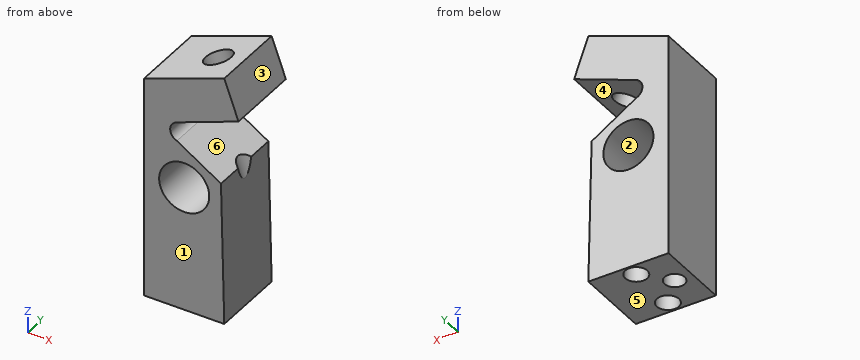
from build123d import *

# Parameters (mm, degrees)
F0_R     = 5
F1_DEPTH = 15
F3_D     = 5.5
F3_DEPTH = 50
F3_TIP   = 1.6523667023
F5_D     = 4.4
F5_DEPTH = 8
F5_TIP   = 1.3218933619
F6_R     = 2
F7_DEPTH = 5


with BuildPart() as f1:
    # F0 (on Front) → F1 (new body)
    with BuildSketch(Plane.XZ):
        with BuildLine():
            Line((-8, -18.9268288441), (8, -18.9268288441))
            Line((8, -18.9268288441), (7.3407884225, 9.531441468))
            Line((7.3407884225, 9.531441468), (-1.4592115775, 15.0849338573))
            ThreePointArc((-1.4592115775, 15.0849338573), (-2.7998378703, 16.9477056406), (-1.5070788684, 18.8440103991))
            Line((-1.5070788684, 18.8440103991), (10.8346573695, 23.5085377897))
            Line((10.8346573695, 23.5085377897), (8, 31.2966949042))
            Line((8, 31.2966949042), (-8, 25.4731711559))
            Line((-8, 25.4731711559), (-8, -18.9268288441))
        make_face()
        with Locations((0, 6.0731711559)):
            Circle(F0_R, mode=Mode.SUBTRACT)
    extrude(amount=F1_DEPTH)

    # F3
    with Locations(Plane(origin=(-9.1227416268, 0, 25.064526623), x_dir=(0.9396926208, 0, 0.3420201433), z_dir=(-0.3420201433, 0, 0.9396926208))):
        with Locations((11.921641043, -7.5)):
            Hole(F3_D / 2, depth=F3_DEPTH)
            with Locations((0, 0, -(F3_DEPTH + F3_TIP / 2))):  # 118° drill point
                Cone(0, F3_D / 2, F3_TIP, mode=Mode.SUBTRACT)

    # F5
    with Locations(Plane(origin=(0, 0, -18.9268288441), x_dir=(1, 0, 0), z_dir=(0, 0, -1))):
        with Locations((0, 12.5), (0, 2.5)):
            Hole(F5_D / 2, depth=F5_DEPTH)
            with Locations((0, 0, -(F5_DEPTH + F5_TIP / 2))):  # 118° drill point
                Cone(0, F5_D / 2, F5_TIP, mode=Mode.SUBTRACT)

    # F6 (on face) → F7 (cut)
    with BuildSketch(Plane(origin=(0, 0, -18.9268288441), x_dir=(1, 0, 0), z_dir=(0, 0, -1))):
        with Locations((-4.5, 7.5)):
            Circle(F6_R)
    extrude(amount=-F7_DEPTH, mode=Mode.SUBTRACT)


solid = f1.part
Part model, mm, in its own coordinate system. Face numbers are marked on the shaded views. A direction names the side the tool comes from. Coordinates: 2 decimals unless noted, no trailing zeros. Order: outer loops, then holes, each group sorted by start corner. A loop starts at its lowest first (then second) coordinate and runs counter-clockwise, first axis right, second up. Notation, with made-up numbers: (-36.5, 34.5) - (22.5, 34.5) arc R25 cw to (22.5, 69.5) - close; hole circle Ø1 at (25.25, 7). An arc over 180 degrees is marked (long way). Use CSV: the item, a comma, the result in double quotes.
Item 1: Saw through at D-D on x = 1.25. Give the number of separate pieces and of enclosed holes in the cut face, and give its area (3 significant figures).
Solved:
separate pieces,"3"
enclosed holes,"0"
area,"392 mm²"
Item 2: Saw through at B-B on x = -4.5. Give the cut face in (y, z).
Solved:
outline,"(-15, -18.93) - (-9.5, -18.93) - (-9.5, -13.93) - (-5.5, -13.93) - (-5.5, -18.93) - (0, -18.93) - (0, 3.89) - (-15, 3.89) - close; (-15, 8.25) - (0, 8.25) - (0, 26.75) - (-15, 26.75) - close"
Item 3: Saw through at A-A on y = -6.5. Give the cut face in (x, z), and give its area (3 significant figures).
Solved:
outline,"(-8, -18.93) - (-6.23, -18.93) - (-6.23, -13.93) - (-2.77, -13.93) - (-2.77, -18.93) - (8, -18.93) - (7.4, 7.04) - (6.24, 10.23) - (-1.46, 15.08) arc R2 cw to (-1.51, 18.84) - (2.54, 20.38) - (-0.33, 28.27) - (-8, 25.47) - close; (4.49, 30.02) - (7.34, 22.19) - (10.83, 23.51) - (8, 31.3) - close; hole circle Ø10 at (0, 6.07)"
area,"536 mm²"
Item 4: Mould opens along Z. For the marked faces 1, 2, 3 and 4 say: +Z half, -Z half, draft (parallel to the pull), parting line (faces both ways), or undercut.
Solved:
face 1,"draft"
face 2,"undercut"
face 3,"+Z half"
face 4,"undercut"
Item 5: Probe probe 1 along Y at (x, z) = (0, -14.5); probe 2 along Y at (x, z) = (-4.5, -17.45); probe 3 along Z at (x, y) = (3, -2). List the from-to ranges inside material, lowest first.
Solved:
probe 1,"y = -15 to -14.7, -10.3 to -4.7, -0.3 to 0"
probe 2,"y = -15 to -9.5, -5.5 to 0"
probe 3,"z = -18.93 to 2.07, 10.07 to 12.27, 20.55 to 29.48"
Item 6: Saw through at C-C on z = 5.5. Give the cut face in (x, y).
Solved:
outline,"(-8, -15) - (-4.97, -15) - (-4.97, 0) - (-8, 0) - close; (4.97, -15) - (7.43, -15) - (7.43, 0) - (4.97, 0) - close"
Item 7: Drop flat-ended pins along their axis: P1, Ø5, axis at y = -2, z = -12.5, coming from the +X side; P2, Ø2.5, axis at x = 0, y = -2.5, coming from the +Z side; P3, Ø10, axis at x = 1, z = 8.5, coming from the -Y side. Give the stop position or say it passes through.
Solved:
P1,"stops at x = 7.91"
P2,"stops at z = 28.84"
P3,"stops at y = -15"
Item 8: 3-axis set-ups, long thin cutter, end or side, ignore diameter. For the marked faces 5 and 6: which of +Z, -Z, +X, -X, +Y, -Y reach the whole face in a straight line?
Solved:
face 5,"-Z, +X, -X, +Y, -Y"
face 6,"+X, +Y, -Y"
